For this review, take the finished solid that the model builds, in its own axes (mm). A direction names the side the tool comes from. Coordinates: 2 decimals unless noted, no trailing zeros. Loops run counter-clockwise (first coordinate to the right, second up) from the corner with the lowest first, then second, coordinate; pieces in that order, holes last.
```python
from build123d import *

# Parameters (mm, degrees)
SKETCH3_R           = 8
BOSS_EXTRUDE3_DEPTH = 5
CUT_EXTRUDE1_DEPTH  = 5
SKETCH6_R           = 4.445
CUT_EXTRUDE2_DEPTH  = 6
SKETCH8_R           = 8
SKETCH8_R_2         = 5.08
BOSS_EXTRUDE4_DEPTH = 10.16


with BuildPart() as part:
    # Sketch3 → Boss-Extrude3 (new body)
    with BuildSketch(Plane(origin=(0, 0, 0), x_dir=(1, 0, 0), z_dir=(0, 1, 0))):
        Circle(SKETCH3_R)
    extrude(amount=BOSS_EXTRUDE3_DEPTH)

    # Sketch4 → Cut-Extrude1 (cut)
    with BuildSketch(Plane(origin=(0, 5, 0), x_dir=(1, 0, 0), z_dir=(0, 1, 0))):
        with BuildLine():
            Line((-0.5999988, 6), (0.5999988, 6))
            ThreePointArc((0.5999988, 6), (0.85189286, 6.99797085), (1.383185318, 7.879517649))
            ThreePointArc((1.383185318, 7.879517649), (0, 8), (-1.383185318, 7.879517649))
            ThreePointArc((-1.383185318, 7.879517649), (-0.85189286, 6.99797085), (-0.5999988, 6))
        make_face()
        with BuildLine():
            Line((2.062722195, 5.66614293), (3.143882674, 5.145483485))
            ThreePointArc((3.143882674, 5.145483485), (3.803834704, 5.935331415), (4.66500149, 6.499058478))
            ThreePointArc((4.66500149, 6.499058478), (3.471069913, 7.207750943), (2.17258767, 7.699341713))
            ThreePointArc((2.17258767, 7.699341713), (2.268776813, 6.674576334), (2.062722195, 5.66614293))
        make_face()
        with BuildLine():
            Line((4.316895762, 4.210036762), (5.065082028, 3.27184086))
            ThreePointArc((5.065082028, 3.27184086), (6.002380434, 3.697126801), (7.022856904, 3.83138107))
            ThreePointArc((7.022856904, 3.83138107), (6.25465186, 4.987918415), (5.298053025, 5.994216725))
            ThreePointArc((5.298053025, 5.994216725), (4.940087414, 5.029200116), (4.316895762, 4.210036762))
        make_face()
        with BuildLine():
            Line((5.71605518, 1.920081181), (5.983079766, 0.750170026))
            ThreePointArc((5.983079766, 0.750170026), (7.012081105, 0.726660882), (7.989749379, 0.404851652))
            ThreePointArc((7.989749379, 0.404851652), (7.799423297, 1.780167472), (7.374174001, 3.1018636))
            ThreePointArc((7.374174001, 3.1018636), (6.632953116, 2.387729136), (5.71605518, 1.920081181))
        make_face()
        with BuildLine():
            Line((5.983079766, -0.750170026), (5.71605518, -1.920081181))
            ThreePointArc((5.71605518, -1.920081181), (6.632953116, -2.387729136), (7.374174001, -3.1018636))
            ThreePointArc((7.374174001, -3.1018636), (7.799423297, -1.780167472), (7.989749379, -0.404851652))
            ThreePointArc((7.989749379, -0.404851652), (7.012081105, -0.726660882), (5.983079766, -0.750170026))
        make_face()
        with BuildLine():
            Line((5.065082028, -3.27184086), (4.316895762, -4.210036762))
            ThreePointArc((4.316895762, -4.210036762), (4.940087414, -5.029200116), (5.298053025, -5.994216725))
            ThreePointArc((5.298053025, -5.994216725), (6.25465186, -4.987918415), (7.022856904, -3.83138107))
            ThreePointArc((7.022856904, -3.83138107), (6.002380434, -3.697126801), (5.065082028, -3.27184086))
        make_face()
        with BuildLine():
            Line((3.143882674, -5.145483485), (2.062722195, -5.66614293))
            ThreePointArc((2.062722195, -5.66614293), (2.268776813, -6.674576334), (2.17258767, -7.699341713))
            ThreePointArc((2.17258767, -7.699341713), (3.471069913, -7.207750943), (4.66500149, -6.499058478))
            ThreePointArc((4.66500149, -6.499058478), (3.803834704, -5.935331415), (3.143882674, -5.145483485))
        make_face()
        with BuildLine():
            Line((0.5999988, -6), (-0.5999988, -6))
            ThreePointArc((-0.5999988, -6), (-0.85189286, -6.99797085), (-1.383185318, -7.879517649))
            ThreePointArc((-1.383185318, -7.879517649), (0, -8), (1.383185318, -7.879517649))
            ThreePointArc((1.383185318, -7.879517649), (0.85189286, -6.99797085), (0.5999988, -6))
        make_face()
        with BuildLine():
            Line((-2.062722195, -5.66614293), (-3.143882674, -5.145483485))
            ThreePointArc((-3.143882674, -5.145483485), (-3.803834704, -5.935331415), (-4.66500149, -6.499058478))
            ThreePointArc((-4.66500149, -6.499058478), (-3.471069913, -7.207750943), (-2.17258767, -7.699341713))
            ThreePointArc((-2.17258767, -7.699341713), (-2.268776813, -6.674576334), (-2.062722195, -5.66614293))
        make_face()
        with BuildLine():
            Line((-4.316895762, -4.210036762), (-5.065082028, -3.27184086))
            ThreePointArc((-5.065082028, -3.27184086), (-6.002380434, -3.697126801), (-7.022856904, -3.83138107))
            ThreePointArc((-7.022856904, -3.83138107), (-6.25465186, -4.987918415), (-5.298053025, -5.994216725))
            ThreePointArc((-5.298053025, -5.994216725), (-4.940087414, -5.029200116), (-4.316895762, -4.210036762))
        make_face()
        with BuildLine():
            Line((-5.71605518, -1.920081181), (-5.983079766, -0.750170026))
            ThreePointArc((-5.983079766, -0.750170026), (-7.012081105, -0.726660882), (-7.989749379, -0.404851652))
            ThreePointArc((-7.989749379, -0.404851652), (-7.799423297, -1.780167472), (-7.374174001, -3.1018636))
            ThreePointArc((-7.374174001, -3.1018636), (-6.632953116, -2.387729136), (-5.71605518, -1.920081181))
        make_face()
        with BuildLine():
            Line((-5.983079766, 0.750170026), (-5.71605518, 1.920081181))
            ThreePointArc((-5.71605518, 1.920081181), (-6.632953116, 2.387729136), (-7.374174001, 3.1018636))
            ThreePointArc((-7.374174001, 3.1018636), (-7.799423297, 1.780167472), (-7.989749379, 0.404851652))
            ThreePointArc((-7.989749379, 0.404851652), (-7.012081105, 0.726660882), (-5.983079766, 0.750170026))
        make_face()
        with BuildLine():
            Line((-5.065082028, 3.27184086), (-4.316895762, 4.210036762))
            ThreePointArc((-4.316895762, 4.210036762), (-4.940087414, 5.029200116), (-5.298053025, 5.994216725))
            ThreePointArc((-5.298053025, 5.994216725), (-6.25465186, 4.987918415), (-7.022856904, 3.83138107))
            ThreePointArc((-7.022856904, 3.83138107), (-6.002380434, 3.697126801), (-5.065082028, 3.27184086))
        make_face()
        with BuildLine():
            Line((-3.143882674, 5.145483485), (-2.062722195, 5.66614293))
            ThreePointArc((-2.062722195, 5.66614293), (-2.268776813, 6.674576334), (-2.17258767, 7.699341713))
            ThreePointArc((-2.17258767, 7.699341713), (-3.471069913, 7.207750943), (-4.66500149, 6.499058478))
            ThreePointArc((-4.66500149, 6.499058478), (-3.803834704, 5.935331415), (-3.143882674, 5.145483485))
        make_face()
    extrude(amount=-CUT_EXTRUDE1_DEPTH, mode=Mode.SUBTRACT)

    # Sketch6 → Cut-Extrude2 (cut, through all)
    with BuildSketch(Plane(origin=(0, 5, 0), x_dir=(1, 0, 0), z_dir=(0, 1, 0))):
        Circle(SKETCH6_R)
    extrude(amount=-CUT_EXTRUDE2_DEPTH, mode=Mode.SUBTRACT)

    # Sketch8 → Boss-Extrude4 (add)
    with BuildSketch(Plane.XZ):
        Circle(SKETCH8_R)
        Circle(SKETCH8_R_2, mode=Mode.SUBTRACT)
    extrude(amount=BOSS_EXTRUDE4_DEPTH)


solid = part.part
```
Q1. Consider section C-C (y = -6.5). State the section outline as (x, z) points.
Q2. Consider section D-D (x = -2.5). State the section outline as (y, z) points, then the cut area to 3 significant figures.
Q3. Wall thickness on probe 1 along X at (y, z) = (2.25, 0) (3 decimals); probe 2 along Z at (x, y) = (0, -4); probe 3 along Z at (x, y) = (0, 2.7) (3 decimals): over which ranges is each line inside the solid? List them lowest first.
Q4. Consider section B-B (x = 6.5). State the section outline as (y, z) points, then the cut area to 3 significant figures.
Q5. Machinability: for faces 4 (the face through (6, 0, 4)), 5 (the face through (0.857, 2.535, 7.011)), 6 (the face through (-6.62, 2.54, -2.38)), which of the approach directions +Z, -Z, +X, -X, +Y, -Y give a long, thin tool a straight path to every point of the face, cutting with its end or side? Answer none if there is none.
Q6. The part is to be moulded in two halves that separate along Z. For faces 1 (the face through (-7, 0, 1)), 2 (the face through (-0.857, 2.535, -7.011)), 3 (the face through (0, 0, -7)), say which applies: +Z half, -Z half, draft (parallel to the pull), parting line (faces both ways), or undercut.
Q7. For pin 1 Ø2 at (x, y) = (6, 0.5) entering from +Z (3 decimals); pin 2 Ø2 at (y, z) = (-3, -5.5) entering from +X; pin 3 Ø0.8 at (x, z) = (3.5, -6.5) entering from +Y, all flat-tipped, find the tip position at first contact; note any pin that passes through.
Q8. Consider section A-A (x = 0). State the section outline as (y, z) points (3 decimals).
Model answer:
1. outline: circle Ø16 at (0, 0); hole circle Ø10.16 at (0, 0)
2. outline: (-10.16, -7.6) - (0, -7.6) - (0, -5.46) - (5, -5.46) - (5, -3.68) - (0, -3.68) - (0, -4.42) - (-10.16, -4.42) - close; (-10.16, 4.42) - (0, 4.42) - (0, 3.68) - (5, 3.68) - (5, 5.46) - (0, 5.46) - (0, 7.6) - (-10.16, 7.6) - close
2. area: 82.4 mm2
3. probe 1: x = -8 to -4.445, 4.445 to 8
3. probe 2: z = -8 to -5.08, 5.08 to 8
3. probe 3: z = -6 to -4.445, 4.445 to 6
4. outline: (-10.16, -4.66) - (0, -4.66) - (0, -3.8) - (5, -3.8) - (5, -2.3) - (0, -2.3) - (0, -0.78) - (5, -0.78) - (5, 0.78) - (0, 0.78) - (0, 2.3) - (5, 2.3) - (5, 3.8) - (0, 3.8) - (0, 4.66) - (-10.16, 4.66) - close
4. area: 118 mm2
5. face 4: +Y
5. face 5: +Z, +Y
5. face 6: -X, +Y
6. face 1: undercut
6. face 2: -Z half
6. face 3: draft
7. pin 1: stops at z = 6.245
7. pin 2: stops at x = 6.61
7. pin 3: stops at y = 0
8. outline: (-10.16, -8) - (0, -8) - (0, -6) - (5, -6) - (5, -4.445) - (0, -4.445) - (0, -5.08) - (-10.16, -5.08) - close; (-10.16, 5.08) - (0, 5.08) - (0, 4.445) - (5, 4.445) - (5, 6) - (0, 6) - (0, 8) - (-10.16, 8) - close
